Read the model definition and answer for the solid it produces. Units are mm, in the model's axes. A direction names the side the tool comes from. Give positions to 0.01 mm unless a question says otherwise; leave off trailing zeros. Order: outer loops, then holes, each group sorted by start corner. A loop starts at its lowest first (then second) coordinate and runs counter-clockwise, first axis right, second up.
Item 1: A cutting plane is placed at D-D (x = 12). Write down the section's boundary in (y, z).
Item 2: Find the intervals of material crossed by line 1 along Y through (x, z) = (7, 0.25); line 2 along Y through (x, z) = (4, 0.45); line 3 along Y through (x, z) = (9, 0.1), in increasing order.
Item 3: A cutting plane is placed at A-A (z = 0.15). Write down the section's boundary in (x, y), plus the area to 3 significant figures.
Item 4: Which of the six approach directions +Z, -Z, +X, -X, +Y, -Y give full straight-line access (tool end or side, diameter ignored) to faces 5 (the face through (14, 4, 0.5)), 6 (the face through (4.776, 2.106, 0.246))?
Item 5: The mould has two halves that part along X. Classify faces 1 (the face through (8.764, 2.106, 0.246)), 2 (the face through (27.761, 2.829, 0.377)), 3 (the face through (14, 4, 0)), 4 (the face through (12.14, 6.13, 0.25)): +X half, -X half, draft (parallel to the pull), parting line (faces both ways), or undercut.
from build123d import *

# Parameters (mm, degrees)
F1_DEPTH    = 0.5
F2_T1_DEPTH = 0.5
F3_W        = 4.74
F3_H        = 2.55
F4_DEPTH    = 0.501
F5_R        = 1.25
F6_SIZE2    = 1.19999
F6_SIZE     = 0.24999


# Not quite as in the source:
# - a fillet or chamfer that OpenCascade refuses, or shapes differently, is made with other operations: its cross-section is extruded or revolved along the edge and cut away or added
# - a fillet or chamfer is up to 0.001 mm smaller than in the source, because OpenCascade refuses the exact size


with BuildPart() as f1:
    # F0 (on Top) → F1 (new body)
    with BuildSketch(Plane.XY):
        Polygon((0, 5.86), (0, 0), (14.7, 0), (14.7, -1.13), (19.8, -1.13), (39.17, 6.9), (14.7, 6.9), (14.7, 5.86), align=None)
    extrude(amount=F1_DEPTH)

    # F2: fillet of radius 14 on 2 edges, made by hand

    # F2_s2 → F2_t1 (join)
    with BuildSketch(Plane.XY):
        with BuildLine():
            ThreePointArc((14.7, 6.9), (12.1030176748, 6.1224601911), (9.4048701621, 5.86))
            Line((9.4048701621, 5.86), (14.7, 5.86))
            Line((14.7, 5.86), (14.7, 6.9))
        make_face()
        with BuildLine():
            ThreePointArc((9.1897277744, 0), (12.0021999965, -0.2854092296), (14.7, -1.13))
            Line((14.7, -1.13), (14.7, 0))
            Line((14.7, 0), (9.1897277744, 0))
        make_face()
    extrude(amount=F2_T1_DEPTH)

    # F3 (on face) → F4 (cut, through all)
    with BuildSketch(Plane.XY.offset(0.5)):
        with Locations((6.77, 3.025)):
            Rectangle(F3_W, F3_H)
    extrude(amount=-F4_DEPTH, mode=Mode.SUBTRACT)

    # F5
    f5_edges = [f1.edges().sort_by_distance(p)[0] for p in [
        (9.14, 1.75, 0.25),
        (4.4, 1.75, 0.25),
        (4.4, 4.3, 0.25),
        (9.14, 4.3, 0.25),
    ]]
    fillet(f5_edges, radius=F5_R)

    # F6 (size 0.25 and 1.2 in the source; OpenCascade refuses exactly that, so slightly less here)
    f6_edges = [f1.edges().sort_by_distance(p)[0] for p in [
        (29.485, 2.885, 0.5),
        (29.485, 2.885, 0),
    ]]
    f6_side = f1.faces().sort_by_distance((29.485, 2.885, 0.25))[0]
    chamfer(f6_edges, length=F6_SIZE, length2=F6_SIZE2, reference=f6_side)


solid = f1.part
Response values:
1. outline: (-0.28, 0) - (6.1, 0) - (6.1, 0.5) - (-0.28, 0.5) - close
2. line 1: y = 0 to 1.75, 4.3 to 5.86
2. line 2: y = 0 to 5.86
2. line 3: y = 0 to 2.43, 3.62 to 5.86
3. outline: (0, 0) - (9.19, 0) arc R14 cw to (14.7, -1.13) - (18.55, -1.13) - (37.92, 6.9) - (14.7, 6.9) arc R14 cw to (9.4, 5.86) - (0, 5.86) - close; hole (4.4, 3) arc R1.25 ccw to (5.65, 1.75) - (7.89, 1.75) arc R1.25 ccw to (9.14, 3) - (9.14, 3.05) arc R1.25 ccw to (7.89, 4.3) - (5.65, 4.3) arc R1.25 ccw to (4.4, 3.05) - close
3. area: 188 mm2
4. face 5: +Z, +X, -X, +Y, -Y
4. face 6: +Z, -Z
5. face 1: undercut
5. face 2: +X half
5. face 3: draft
5. face 4: -X half
